Geometry check sheet. Reference: the model listing, model coordinates, mm. A direction names the side the tool comes from. Give positions to 0.01 mm unless a question says otherwise; leave off trailing zeros. Order: outer loops, then holes, each group sorted by start corner. A loop starts at its lowest first (then second) coordinate and runs counter-clockwise, first axis right, second up. Notation, with made-up numbers: (60, 64.25) - (68, 64.25) arc R11 cw to (68, 70.25) - close; hole circle Ø10 at (-10.75, 49.25). An arc over 180 degrees is marked (long way). Put each result on its own line as item: value. Start each with the question number.
```python
from build123d import *

# Parameters (mm, degrees)
SKETCH_1_R          = 25
EXTRUDE_1_DEPTH     = 5
SKETCH_4_W          = 14.5
SKETCH_4_H          = 1
SKETCH_5_R          = 1
CUT_EXTRUDE_3_DEPTH = 36.707142143


with BuildPart() as part:
    # 草图1 → 凸台-拉伸1 (new body)
    with BuildSketch(Plane(origin=(0, 0, 0), x_dir=(1, 0, 0), z_dir=(0, 1, 0))):
        with Locations(Location((0, 0, 0), (0, 0, 270))):
            Circle(SKETCH_1_R)
    extrude(amount=EXTRUDE_1_DEPTH)

    # 草图4 → 切除-旋转1 (revolve, cut)
    with BuildSketch(Plane.XY, mode=Mode.PRIVATE) as cut_revolve_1_sk:
        with Locations((7.25, 4.5)):
            Rectangle(SKETCH_4_W, SKETCH_4_H)
        Polygon((18.5, 1.5), (18.5, 5), (14.5, 5), (14.5, 4), align=None)
    revolve(cut_revolve_1_sk.sketch.rotate(Axis((0, 0, 0), (0, 1, 0)), 90), axis=Axis((0, 0, 0), (0, 1, 0)), mode=Mode.SUBTRACT)

    # 草图5 → 切除-拉伸3 (cut, through all)
    with BuildSketch(Plane(origin=(0, 5, 0), x_dir=(1, 0, 0), z_dir=(0, 1, 0))):
        with Locations(Location((0, 23, 0), (0, 0, 270))):
            Circle(SKETCH_5_R)
        with Locations(Location((23, 0, 0), (0, 0, 270))):
            Circle(SKETCH_5_R)
        with Locations(Location((0, -23, 0), (0, 0, 270))):
            Circle(SKETCH_5_R)
        with Locations(Location((-23, 0, 0), (0, 0, 270))):
            Circle(SKETCH_5_R)
    extrude(amount=-CUT_EXTRUDE_3_DEPTH, mode=Mode.SUBTRACT)


solid = part.part
```
Item 1: Gauge pin test, flat ends, axial feed: pin 1 Ø1 at (x, y) = (-1, 2.5) entering from -Z (3 decimals); pin 2 Ø1.2 at (x, z) = (23, 0) entering from +Y; pin 3 Ø3 at (x, z) = (-9.5, -5) entering from +Y; pin 4 Ø2 at (y, z) = (3.5, 16.5) entering from +X. Record the tip position at first contact, or that the pin passes through.
Item 2: Cross-section at B-B (z = 23). Enter the section's corners in (x, y).
Item 3: Release check for a two-part mould opening along X. For faces 1 (the face through (-18.4, 5, -3.8)), 2 (the face through (7.509, 2.465, 23.846)), 3 (the face through (0, 3, -24)) record: +X half, -X half, draft (parallel to the pull), parting line (faces both ways), or undercut.
Item 4: Set-up check for faces 4 (the face through (-24, 3, 0)), 5 (the face through (0, 4, 0)): record each of +Z, -Z, +X, -X, +Y, -Y from which the full face is reachable in a straight line by a thin tool's end or side.
Item 5: Cross-section at C-C (x = -23). Enter the section's corners in (y, z).
Item 6: Cross-section at A-A (z = 0). Enter the section's corners in (x, y), and give its area (3 significant figures).
Item 7: Thickness scan on line 1 along X through (y, z) = (1.1, 0); line 2 along X through (y, z) = (1.8, 0); line 3 along X through (y, z) = (2.8, 0). Record the ranges inside material, lowest first.
Recorded:
1. pin 1: stops at z = -24.995
1. pin 2: passes through
1. pin 3: stops at y = 4
1. pin 4: stops at x = 19.62
2. outline: (-9.8, 0) - (-1, 0) - (-1, 5) - (-9.8, 5) - close; (1, 0) - (9.8, 0) - (9.8, 5) - (1, 5) - close
3. face 1: draft
3. face 2: parting line
3. face 3: undercut
4. face 4: +Y, -Y
4. face 5: +Y
5. outline: (0, -9.8) - (5, -9.8) - (5, -1) - (0, -1) - close; (0, 1) - (5, 1) - (5, 9.8) - (0, 9.8) - close
6. outline: (-25, 0) - (-24, 0) - (-24, 5) - (-25, 5) - close; (-22, 0) - (22, 0) - (22, 5) - (18.5, 5) - (18.5, 1.5) - (14.5, 4) - (-14.5, 4) - (-18.5, 1.5) - (-18.5, 5) - (-22, 5) - close; (24, 0) - (25, 0) - (25, 5) - (24, 5) - close
6. area: 183 mm^2
7. line 1: x = -25 to -24, -22 to 22, 24 to 25
7. line 2: x = -25 to -24, -22 to -18.5, -18.02 to 18.02, 18.5 to 22, 24 to 25
7. line 3: x = -25 to -24, -22 to -18.5, -16.42 to 16.42, 18.5 to 22, 24 to 25
